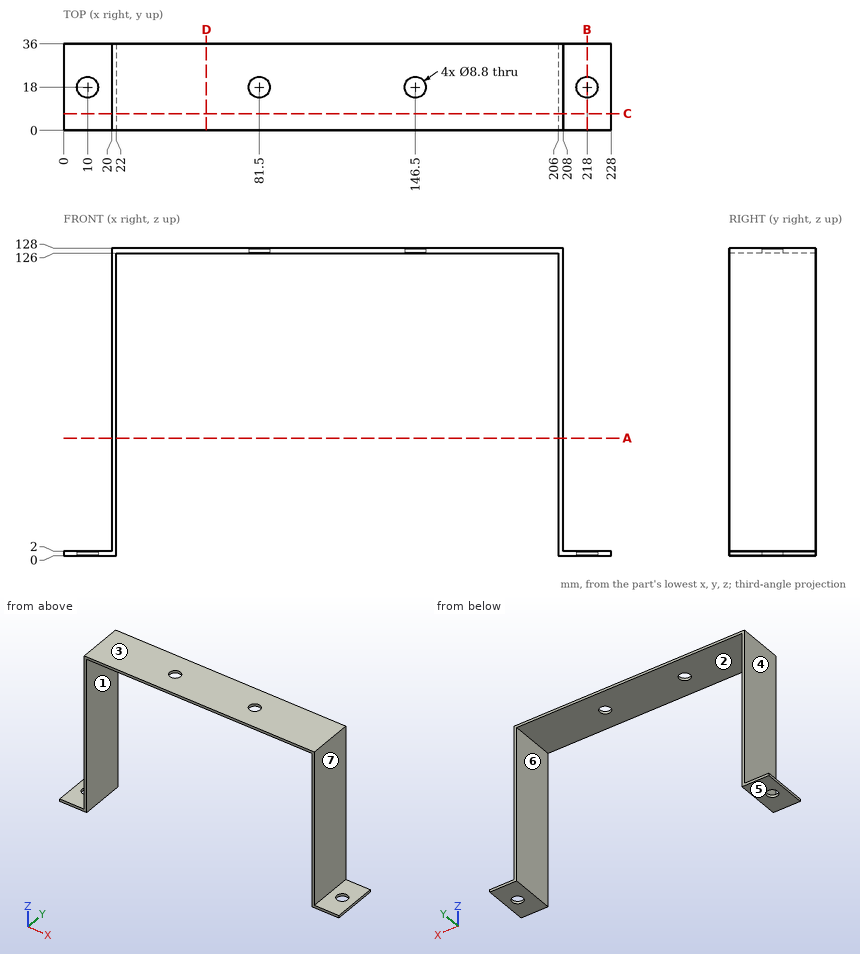
Input: dimensioned drawing with shaded views. Units: mm. Origin: part minimum x, y, z. A direction names the side the tool comes from. Give positions to 0.01 mm unless a question says otherwise; leave off trailing zeros. Write each loop counter-clockwise with the first axis right and the second up, starting at its lowest first coordinate (ties: lowest second). Pieces come first, ordered by that corner, then holes.
Q1. Set-up query: the marked faces 5, 6 and 7. Return all of +Z, -Z, +X, -X, +Y, -Y with unobstructed straight access to the full face (end or side cutting, diameter ignored); none if empty.
Q2. Section A-A, the plane z = 49. Output: boundary loops of the cut face in (x, y).
Q3. Section D-D, the plane x = 59.5. Output: boundary loops of the cut face in (y, z).
Q4. Material intervals for probe 1 along Y at (x, z) = (81.5, 127.65); probe 2 along X at (y, z) = (28, 111.5); probe 3 along Z at (x, y) = (57.5, 2), sorted ascending.
Q5. First-contact query: P1, Ø1, axis at x = 99, y = 30.5, coming from the -Z side; P2, Ø18, axis at y = 17.5, z = 88.5, coming from the +X side; P3, Ø11.5, axis at x = 10, y = 18, coming from the +Z side; P4, Ø10, axis at x = 218, y = 18, coming from the -Z side. Flat tips, straight axial feed; report the tip coordinate or a pass-through.
Q6. Pull-direction query (X, two-part tool) for the marked faces 1, 2, 3 and 4; classes: pulls with the +X half, pulls with the -X half, needs draft (parallel to the pull), parting line crosses it, or undercut.
Q7. Section C-C, the plane y = 7. Output: boundary loops of the cut face in (x, z).
Q8. Section B-B, the plane x = 218. Output: boundary loops of the cut face in (y, z), plus the area to 3 significant figures.
Filled in:
1. face 5: -Z, +X, -X, +Y, -Y
1. face 6: -Z, +Y, -Y
1. face 7: +Z, +X, +Y, -Y
2. outline: (20, 0) - (22, 0) - (22, 36) - (20, 36) - close; (206, 0) - (208, 0) - (208, 36) - (206, 36) - close
3. outline: (0, 126) - (36, 126) - (36, 128) - (0, 128) - close
4. probe 1: y = 0 to 13.6, 22.4 to 36
4. probe 2: x = 20 to 22, 206 to 208
4. probe 3: z = 126 to 128
5. P1: stops at z = 126
5. P2: stops at x = 208
5. P3: stops at z = 2
5. P4: stops at z = 0
6. face 1: undercut
6. face 2: undercut
6. face 3: needs draft
6. face 4: pulls with the -X half
7. outline: (0, 0) - (22, 0) - (22, 126) - (206, 126) - (206, 0) - (228, 0) - (228, 2) - (208, 2) - (208, 128) - (20, 128) - (20, 2) - (0, 2) - close
8. outline: (0, 0) - (13.6, 0) - (13.6, 2) - (0, 2) - close; (22.4, 0) - (36, 0) - (36, 2) - (22.4, 2) - close
8. area: 54.4 mm2
